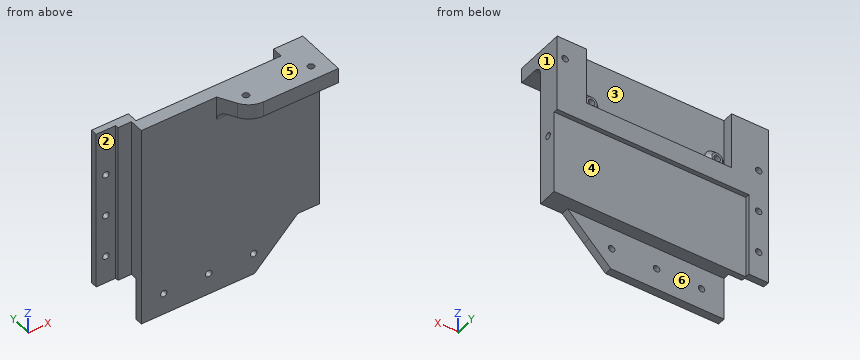
Autodesk Inventor part; units mm, degrees
ref_plane "YZ Plane" through (0, 0, 0) normal (1, 0, 0) x (0, 1, 0)
ref_plane "XZ Plane" through (0, 0, 0) normal (0, 1, 0) x (-1, 0, 0)
ref_plane "XY Plane" through (0, 0, 0) normal (0, 0, 1) x (1, 0, 0)
sketch "Sketch1" plane through (0, 0, 0) normal (0, 0, 1) x (1, 0, 0)
  line L0 (-48.75, -5.5) -> (48.75, -5.5)
  line L1 (48.75, -5.5) -> (48.75, 5.5)
  line L2 (48.75, 5.5) -> (-48.75, 5.5)
  line L3 (-48.75, 5.5) -> (-48.75, -5.5)
  line L4 (-48.75, -5.5) -> (48.75, 5.5) construction
  line L5 (48.75, -5.5) -> (-48.75, 5.5) construction
  line L6 (-48.75, 2.5) -> (-39.75, 2.5)
  line L7 (-39.75, 2.5) -> (-39.75, 1)
  line L8 (-39.75, 1) -> (-33.5, 1)
  line L9 (-33.5, 1) -> (-33.5, -5.5)
  point P0 (0, 0)
  dimension "d0" = 11
  dimension "d1" = 97.5
  dimension "d2" = 9
  dimension "d3" = 6.25
  dimension "d4" = 1.5
  dimension "d5" = 6.5
extrude "Extrusion1" add sketch "Sketch1" along normal blind 75 contours L9 L8 L7 L6 L3 L2 L1 L0
sketch "Sketch2" plane through (-48.75, 2.5, 0) normal (0, -1, 0) x (1, 0, 0)
  line L0 (0, 0) -> (9, 0)
  point P0 (48.75, 0)
  point P1 (4.5, 13)
  point P2 (4.5, 33)
  point P3 (4.5, 53)
  point P4 (4.5, 0)
  point P5 (4.5, 0)
  point P6 (4.5, 73)
  dimension "d8" = 13
  dimension "d9" = 20
  dimension "d10" = 20
  dimension "d11" = 20
hole "Hole1" at (-44.25, 2.5, 13) at (-44.25, 2.5, 33) at (-44.25, 2.5, 53) direction (0, 1, 0) diameter 3 depth 15
sketch "Sketch3" plane through (48.75, -5.5, 0) normal (1, 0, 0) x (0, 0, -1)
  line L0 (0, 0) -> (0, 11)
  line L1 (0, 11) -> (-75, 11)
  line L2 (-75, 0) -> (-75, 11)
  line L3 (0, 0) -> (-75, 0)
  point P0 (0, 5.5)
  point P1 (-30, 5)
  point P2 (0, 5.5)
  dimension "d19" = 30
  dimension "d20" = 5
hole "Hole2" at (48.75, -0.5, 30) direction (-1, 0, 0) diameter 3 depth 15
sketch "Sketch4" plane through (-33.5, -5.5, 0) normal (0, -1, 0) x (1, 0, 0)
  line L0 (0, 0) -> (82.25, 0)
  line L1 (82.25, 0) -> (82.25, 75)
  line L2 (0, 75) -> (82.25, 75)
  line L3 (0, 0) -> (0, 75)
  line L4 (0, 0) -> (0, -20)
  line L5 (0, -20) -> (62.25, -20)
  line L6 (62.25, -20) -> (62.25, 0)
  point P0 (33.5, 0)
  dimension "d28" = 20
  dimension "d29" = 20
extrude "Extrusion2" add sketch "Sketch4" against normal blind 3.5 contours L0 L6 L5 L4
chamfer "Chamfer1" distance 10 angle 45 2 edges at (28.75, -3.75, -20) (28.75, -3.75, 0)
sketch "Sketch5" plane through (-33.5, -5.5, 75) normal (0, -1, 0) x (1, 0, 0)
  line L0 (0, -95) -> (0, 0)
  line L1 (0, -95) -> (52.25, -95)
  line L2 (62.25, -75) -> (0, -75)
  line L3 (62.25, -75) -> (62.25, -95)
  line L4 (62.25, -95) -> (52.25, -95)
  point P0 (33.5, -75)
  point P1 (10.375, -85)
  point P2 (31.125, -85)
  point P3 (51.875, -85)
  dimension "d36" = 10.375
  dimension "d37" = 20.75
  dimension "d38" = 20.75
  dimension "d39" = 20
  dimension "d40" = 10
hole "Hole3" at (-23.125, -5.5, -10) at (-2.375, -5.5, -10) at (18.375, -5.5, -10) direction (0, 1, 0) diameter 3 depth 15
sketch "Sketch6" plane through (0, 0, 75) normal (0, 0, 1) x (1, 0, 0)
  line L0 (-33.5, -5.5) -> (48.75, -5.5)
  line L1 (48.75, -5.5) -> (48.75, -18)
  line L2 (48.75, -18) -> (8.5, -18)
  line L3 (8.5, -18) -> (-56.5, 94.5833)
  line L4 (-56.5, 94.5833) -> (-56.5, 62)
  point P0 (0, 0)
  point P1 (48.75, -11.75)
  point P2 (1.2831, -5.5)
  dimension "d48" = 12.5
  dimension "d49" = 120
  dimension "d50" = 105.25
  dimension "d51" = 80
  dimension "d52" = 65
extrude "Extrusion3" add sketch "Sketch6" against normal blind 7
fillet "Fillet1" radius 4 1 edges at (25.0166, -5.5, 68)
fillet "Fillet2" radius 10 1 edges at (8.5, -18, 71.5)
sketch "Sketch7" plane through (0, 0, 75) normal (0, 0, 1) x (1, 0, 0)
  arc A0 (5.6132, -13) -> (14.2735, -18) centre (14.2735, -8) ccw
  line L0 (14.2735, -18) -> (48.75, -18)
  line L1 (48.75, -18) -> (48.75, 5.5)
  line L2 (48.75, 5.5) -> (-48.75, 5.5)
  line L3 (-48.75, 5.5) -> (-48.75, 2.5)
  line L4 (-48.75, 2.5) -> (-39.75, 2.5)
  line L5 (-39.75, 2.5) -> (-39.75, 1)
  line L6 (-39.75, 1) -> (-33.5, 1)
  line L7 (-33.5, 1) -> (-33.5, -5.5)
  line L8 (-33.5, -5.5) -> (1.2831, -5.5)
  line L9 (1.2831, -5.5) -> (5.6132, -13)
  point P0 (0, 0)
  point P1 (41, -11)
  point P2 (11, -11)
  dimension "d57" = 30
  dimension "d58" = 7.75
  dimension "d59" = 7
hole "Hole4" at (41, -11, 75) at (11, -11, 75) direction (0, 0, -1) diameter 3 depth 15
sketch "Sketch8" plane through (-48.75, 5.5, 0) normal (0, 1, 0) x (1, 0, 0)
  line L0 (97.5, -75) -> (0, -75)
  line L1 (97.5, 0) -> (97.5, -75)
  point P0 (48.75, 0)
  point P1 (93.875, -65.5)
  dimension "d67" = 9.5
  dimension "d68" = 3.625
hole "Hole5" at (45.125, 5.5, 65.5) direction (0, -1, 0) diameter 3 depth 10
sketch "Sketch9" plane through (-48.75, 5.5, 0) normal (0, 1, 0) x (1, 0, 0)
  line L0 (18, -79.5) -> (83, -79.5)
  line L1 (83, -79.5) -> (83, -49.5)
  line L2 (83, -49.5) -> (18, -49.5)
  line L3 (18, -49.5) -> (18, -79.5)
  line L4 (18, -79.5) -> (83, -49.5) construction
  line L5 (83, -79.5) -> (18, -49.5) construction
  line L6 (21.5, -76) -> (79.5, -76)
  line L7 (79.5, -76) -> (79.5, -53)
  line L8 (79.5, -53) -> (21.5, -53)
  line L9 (21.5, -53) -> (21.5, -76)
  line L10 (21.5, -76) -> (79.5, -53) construction
  line L11 (79.5, -76) -> (21.5, -53) construction
  line L12 (97.5, -75) -> (0, -75)
  line L13 (97.5, 0) -> (97.5, -75)
  line L14 (17, -48.5) -> (84, -48.5)
  line L15 (84, -48.5) -> (84, -80.5)
  line L16 (84, -80.5) -> (17, -80.5)
  line L17 (17, -80.5) -> (17, -48.5)
  point P0 (48.75, 0)
  point P1 (50.5, -64.5)
  point P2 (83, -75)
  point P3 (84, -75)
  point P4 (17, -75)
  point P5 (18, -75)
  dimension "d76" = 65
  dimension "d77" = 30
  dimension "d78" = 58
  dimension "d79" = 23
  dimension "d80" = 47
  dimension "d97" = 4.5
  dimension "d103" = 1
extrude "Extrusion4" cut sketch "Sketch9" against normal blind 5 contours L3 L12 L9 L6 L7 L1 L0 | L12 L17 L14 L15 L1 L2 L3 | L3 L2 L1 L12 L7 L8 L9 | L12 L7 L6 L9 | L9 L8 L7 L12
hole "Hole6" at (30.75, 5.5, 53) at (-27.25, 5.5, 53) direction (0, -1, 0) diameter 3 depth 10
sketch "Sketch10" plane through (-48.75, 0.5, 0) normal (0, 1, 0) x (1, 0, 0)
  circle A0 centre (21.5, -53) radius 1.5
  circle A1 centre (79.5, -53) radius 1.5
  line L0 (84, -75) -> (17, -75)
  circle A2 centre (21.5, -53) radius 2.5
  circle A3 centre (79.5, -53) radius 2.5
  circle A4 centre (76.5, -76) radius 2.5
  circle A5 centre (18.5, -76) radius 2.5
  line L1 (84, -48.5) -> (84, -75)
  line L2 (17, -48.5) -> (84, -48.5)
  line L3 (17, -75) -> (17, -48.5)
  point P0 (48.75, 0)
  point P1 (78.7913, -75)
  point P2 (74.2087, -75)
  point P3 (20.7913, -75)
  point P4 (20.7913, -75)
  dimension "d91" = 1
extrude "Extrusion5" add sketch "Sketch10" along normal blind 2 contours A2 | A3
chamfer "Chamfer2" distance 2 angle 45 2 edges at (28.25, 0.5, 53) (-29.75, 0.5, 53)
sketch "Sketch11" plane through (-48.75, 5.5, 0) normal (0, 1, 0) x (1, 0, 0)
  line L0 (97.5, -75) -> (84, -75)
  line L1 (97.5, 0) -> (97.5, -75)
  line L2 (97.5, 0) -> (0, 0)
  line L3 (0, 0) -> (0, -75)
  line L4 (17, -75) -> (0, -75)
  circle A0 centre (93.875, -65.5) radius 1.5
  circle A1 centre (4.5, -53) radius 1.5
  circle A2 centre (4.5, -33) radius 1.5
  circle A3 centre (4.5, -13) radius 1.5
  line L5 (9, 0.062) -> (9, -75.3378)
  line L6 (0, -39) -> (97.5, -39)
  line L7 (84, -48.5) -> (84, -75)
  line L8 (17, -75) -> (17, -48.5)
  line L9 (17, -48.5) -> (84, -48.5)
  point P0 (48.75, 0)
  point P1 (90.75, -75)
  point P2 (9, -39)
  point P3 (9, 0)
  dimension "d99" = 9
  dimension "d100" = 36
extrude "Extrusion6" cut sketch "Sketch11" against normal blind 2 contours L6 L5 L2 L1
properties part number "BottomSlideMountExtension" material "ABS Plastic"
Work out the finished part from the listing and answer in its coordinate system (mm). Face numbers are marked on the shaded views. A direction names the side the tool comes from. Give positions to 0.01 mm unless a question says otherwise; leave off trailing zeros. Write each loop counter-clockwise with the first axis right and the second up, starting at its lowest first coordinate (ties: lowest second). Pieces come first, ordered by that corner, then holes.
Q1. The part is cut by section A-A on z = 13. Give the vertices of the cut face in (x, y).
Answer:
outline: (-48.75, 2.5) - (-45.75, 2.5) - (-45.75, 5.5) - (-48.75, 5.5) - close; (-42.75, 2.5) - (-39.75, 2.5) - (-39.75, 1) - (-33.5, 1) - (-33.5, -5.5) - (48.75, -5.5) - (48.75, 3.5) - (-39.75, 3.5) - (-39.75, 5.5) - (-42.75, 5.5) - close
Q2. The part is cut by section C-C on x = -15. Give the vertices of the cut face in (y, z), and give its area (4 significant figures).
Answer:
outline: (-5.5, -20) - (-2, -20) - (-2, 0) - (3.5, 0) - (3.5, 39) - (5.5, 39) - (5.5, 48.5) - (0.5, 48.5) - (0.5, 75) - (-5.5, 75) - close
area: 684.5 mm2
Q3. A tool of negligible diameter and unlimited length cuts with its end or side. For the marked faces 4, 5 and 6, from which of +Z, -Z, +X, -X, +Y, -Y can it reach the whole face along a straight path? Write none if from no direction.
Answer:
face 4: -Z, +X, +Y
face 5: +Z, +X, -X, +Y, -Y
face 6: -Z, +X, -X, +Y
Q4. For a pull along X with two mould halves and no side action, classify the marked faces 1, 2 and 3 as released by +X, released by -X, zero draft, split by the parting line, or undercut.
Answer:
face 1: released by +X
face 2: zero draft
face 3: undercut
Q5. Straight lines are drawn through the part: L1, parallel to X at y = 4.5, z = 53; L2, parallel to Y at x = 41, z = 30; L3, parallel to X at y = 3.2, z = 33. For each, find the intervals that lie inside material, in ascending order.
Answer:
L1: x = -48.75 to -45.75, -42.75 to -31.75, 35.25 to 48.75
L2: y = -5.5 to -2, 1 to 3.5
L3: x = -48.75 to -45.75, -42.75 to 48.75
Q6. The part is cut by section D-D on z = 30. Give the vertices of the cut face in (x, y).
Answer:
outline: (-48.75, 2.5) - (-39.75, 2.5) - (-39.75, 1) - (-33.5, 1) - (-33.5, -5.5) - (48.75, -5.5) - (48.75, -2) - (33.75, -2) - (33.75, 1) - (48.75, 1) - (48.75, 3.5) - (-39.75, 3.5) - (-39.75, 5.5) - (-48.75, 5.5) - close
Q7. The part is cut by section B-B on y = -11. Give the vertices of the cut face in (x, z), and give its area (3 significant figures).
Answer:
outline: (4.46, 68) - (9.5, 68) - (9.5, 75) - (4.46, 75) - close; (12.5, 68) - (39.5, 68) - (39.5, 75) - (12.5, 75) - close; (42.5, 68) - (48.75, 68) - (48.75, 75) - (42.5, 75) - close
area: 268 mm2
Q8. Given pin 1 (7 mm diameter, centred on x = -36, z = 51.5, fed in from -Y); pin 2 (2.5 mm diameter, centred on x = 20, y = -13.5, fed in from -Z); pin 3 (10 mm diameter, centred on x = -9, z = -8, fed in from +Y), each flat-ended and moving along its own axis, determine where each tip first touches the part or whether it passes through.
Answer:
pin 1: stops at y = -5.5
pin 2: stops at z = 68
pin 3: stops at y = -2
